Build history of the part. All positions in model axes, mm. A direction names the side the tool comes from. Coordinates: 2 decimals unless noted, no trailing zeros. Order: outer loops, then holes, each group sorted by start corner. A loop starts at its lowest first (then second) coordinate and runs counter-clockwise, first axis right, second up. Notation, with made-up numbers: (-10.75, -22.5) -> (42.25, -22.5) arc R18 cw to (42.25, 2.5) -> close; hole circle Ø2 at (20.25, 23.5). An arc over 180 degrees is marked (long way). Write each question's results on one line, items separated by ' | '.
from build123d import *

# Parameters (mm, degrees)
SKETCH1_W                    = 13
SKETCH1_H                    = 25
BASE_FLANGE1_DEPTH           = 0.86
EDGE_FLANGE1_STRIP_W         = 4.9132
EDGE_FLANGE1_STRIP_H         = 0.86
EDGE_FLANGE1_STRIP_CUT_DEPTH = 13
EDGE_FLANGE1_DEPTH           = 13
FILLET1_R                    = 2
SKETCH10_R                   = 1.55
CUT_EXTRUDE1_DEPTH           = 22.112546033
CUT_EXTRUDE2_DEPTH           = 30.870554062


# Sheet-metal steps are written as plain solids
with BuildPart() as part:
    # Sketch1 → Base-Flange1 (new body)
    with BuildSketch(Plane(origin=(0, 0, 0), x_dir=(1, 0, 0), z_dir=(0, 1, 0))):
        Rectangle(SKETCH1_W, SKETCH1_H)
    extrude(amount=-BASE_FLANGE1_DEPTH)

    # Edge-Flange1 strip (across the edge) → Edge-Flange1 strip cut (cut)
    with BuildSketch(Plane(origin=(-6.5, 0, 12.5), x_dir=(0, 0, -1), z_dir=(1, 0, 0))):
        with Locations((-1.72, -0.43)):
            Rectangle(EDGE_FLANGE1_STRIP_W, EDGE_FLANGE1_STRIP_H)
    extrude(amount=EDGE_FLANGE1_STRIP_CUT_DEPTH, mode=Mode.SUBTRACT)

    # Edge-Flange1 section (across the edge) → Edge-Flange1 (add)
    with BuildSketch(Plane(origin=(-6.5, 0, 12.5), x_dir=(0, 0, -1), z_dir=(1, 0, 0))):
        with BuildLine():
            Line((-0.86, 0.7366), (-0.86, 15))
            Line((-0.86, 15), (0, 15))
            Line((0, 15), (0, 0.7366))
            ThreePointArc((0, 0.7366), (0.215745145, 0.215745145), (0.7366, 0))
            Line((0.7366, 0), (0.7366, -0.86))
            ThreePointArc((0.7366, -0.86), (-0.392366687, -0.392366687), (-0.86, 0.7366))
        make_face()
    extrude(amount=EDGE_FLANGE1_DEPTH)

    # Fillet1
    fillet1_edges = [part.edges().sort_by_distance(p)[0] for p in [
        (-6.5, 15, 12.93),
        (6.5, 15, 12.93),
        (-6.5, -0.43, -12.5),
        (6.5, -0.43, -12.5),
    ]]
    fillet(fillet1_edges, radius=FILLET1_R)

    # Sketch10 → Cut-Extrude1 (cut, through all)
    with BuildSketch(Plane(origin=(0, 0, 0), x_dir=(1, 0, 0), z_dir=(0, 1, 0))):
        with Locations(Location((0, 6.7, 0), (0, 0, 270))):
            Circle(SKETCH10_R)
    extrude(amount=-CUT_EXTRUDE1_DEPTH, mode=Mode.SUBTRACT)

    # Sketch11 → Cut-Extrude2 (cut, through all)
    with BuildSketch(Plane(origin=(0, 0, 12.5), x_dir=(-1, 0, 0), z_dir=(0, 0, -1))):
        with BuildLine():
            Line((1.7, 9), (1.7, 6.7366))
            ThreePointArc((1.7, 6.7366), (0, 5.0366), (-1.7, 6.7366))
            Line((-1.7, 6.7366), (-1.7, 9))
            ThreePointArc((-1.7, 9), (0, 10.7), (1.7, 9))
        make_face()
    extrude(amount=-CUT_EXTRUDE2_DEPTH, mode=Mode.SUBTRACT)


solid = part.part
Item 1: Pull direction Y, two halves, no side cores. Call faces 1 (the flat face through (-1.7, 8, 13)), 2 (the flat face through (-6.5, -0.6, 4.9)), 3 (the cylindrical face through (-0.091, -0.405, 12.88)): released by +Y, released by -Y, zero draft, split by the parting line, or undercut.
Answer:
face 1: undercut | face 2: zero draft | face 3: released by -Y
Item 2: Slice it at A-A, the plane x = 0. List the corners of the cut face in (y, z), and give its area (3 significant figures).
Answer:
outline: (-0.86, -12.5) -> (0, -12.5) -> (0, -8.25) -> (-0.86, -8.25) -> close; (-0.86, -5.15) -> (0, -5.15) -> (0, 11.76) arc R0.74 cw to (0.74, 12.5) -> (5.04, 12.5) -> (5.04, 13.36) -> (0.74, 13.36) arc R1.6 ccw to (-0.86, 11.76) -> close; (10.7, 12.5) -> (15, 12.5) -> (15, 13.36) -> (10.7, 13.36) -> close | area: 27.2 mm^2
Item 3: Pin check, flat tips, straight feed: pin 1 (6.5 mm diameter, centred on x = 0.5, z = 4.5, fed in from +Y); pin 2 (2 mm diameter, centred on x = 0, y = 4, fed in from -Z). Stop position of each tip, or through.
Answer:
pin 1: stops at y = 0 | pin 2: stops at z = 12.5
Item 4: Slice it at B-B, the plane y = 5.75. List the corners of the cut face in (x, z).
Answer:
outline: (-6.5, 12.5) -> (-1.38, 12.5) -> (-1.38, 13.36) -> (-6.5, 13.36) -> close; (1.38, 12.5) -> (6.5, 12.5) -> (6.5, 13.36) -> (1.38, 13.36) -> close
Item 5: Drill centre lines: line 1 (X direction, y = -0.5, z = -6.7); line 2 (Y direction, x = -1.75, z = 8); line 3 (Z direction, x = 2.25, y = 7.5). Where is each one in solid material? Low to high. Write a range as from..to.
Answer:
line 1: x = -6.5..-1.55, 1.55..6.5 | line 2: y = -0.86..0 | line 3: z = 12.5..13.36
Item 6: Slice it at C-C, the plane z = -6.7. List the corners of the cut face in (x, y), and give its area (3 significant figures).
Answer:
outline: (-6.5, -0.86) -> (-1.55, -0.86) -> (-1.55, 0) -> (-6.5, 0) -> close; (1.55, -0.86) -> (6.5, -0.86) -> (6.5, 0) -> (1.55, 0) -> close | area: 8.51 mm^2
Item 7: Slice it at D-D, the plane x = -4. List the corners of the cut face in (y, z).
Answer:
outline: (-0.86, -12.5) -> (0, -12.5) -> (0, 11.76) arc R0.74 cw to (0.74, 12.5) -> (15, 12.5) -> (15, 13.36) -> (0.74, 13.36) arc R1.6 ccw to (-0.86, 11.76) -> close
Item 8: Tool access for faces 4 (the cylindrical face through (-0.037, 5.037, 12.924)), 5 (the flat face through (0, 15, 13)), 6 (the flat face through (0, 0, -1)): list every direction of +Z, -Z, +X, -X, +Y, -Y with a clear straight run to the whole face (end or side of a thin tool).
Answer:
face 4: +Z, -Z | face 5: +Z, -Z, +X, -X, +Y | face 6: -Z, +X, -X, +Y
